Design review of the part shown in the three views and the two pictorial views. Dimensions are in mm from the part's minimum x, y and z. A direction names the side the tool comes from. Give positions to 0.01 mm unless a question says otherwise; leave off trailing zeros. Loops run counter-clockwise (first coordinate to the right, second up) from the corner with the lowest first, then second, coordinate; pieces in that order, holes last.
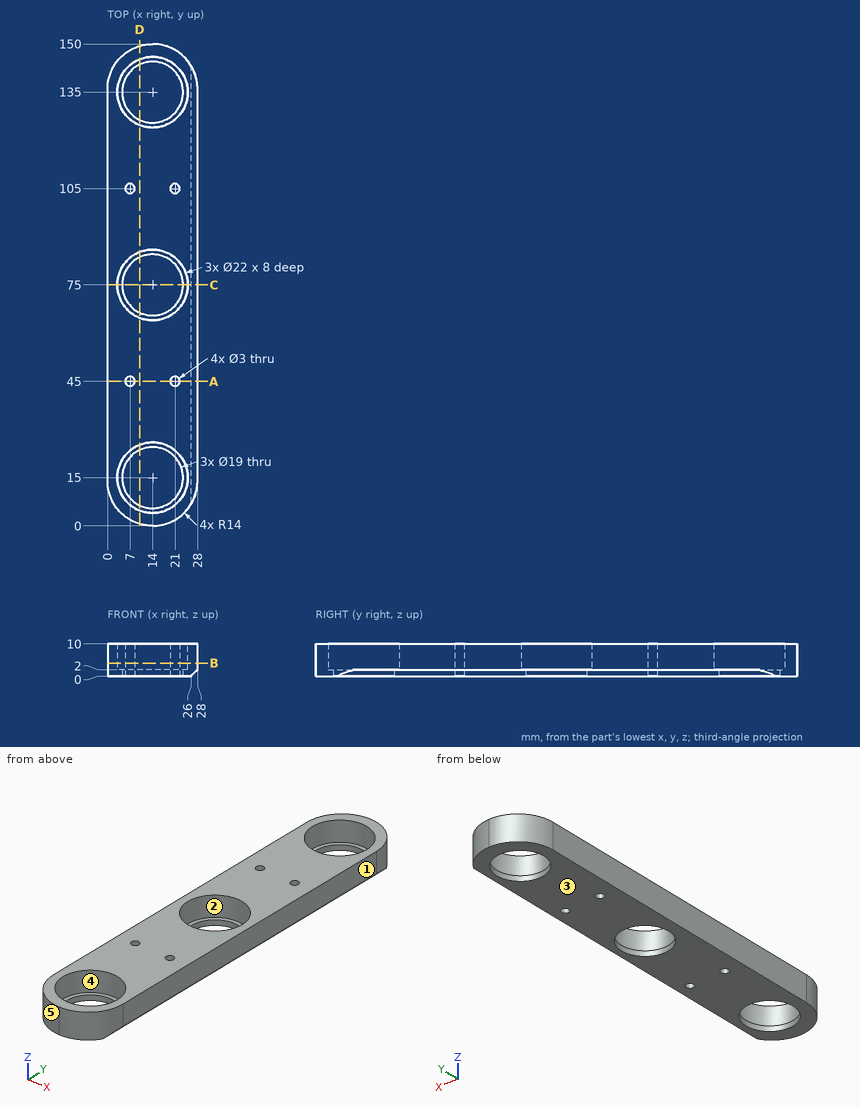
Q1. For probe 1 along X at (y, z) = (45, 6.25); probe 2 along Y at (x, z) = (14, 0.6); probe 3 along Y at (x, z) = (7, 4) (1 decimal), list the stretches that pass through material, from the lowest coordinate up.
Answers:
probe 1: x = 0 to 5.5, 8.5 to 19.5, 22.5 to 28
probe 2: y = 0 to 5.5, 24.5 to 65.5, 84.5 to 125.5, 144.5 to 150
probe 3: y = 1.9 to 6.5, 23.5 to 43.5, 46.5 to 66.5, 83.5 to 103.5, 106.5 to 126.5, 143.5 to 148.1
Q2. Consider section C-C on y = 75. Give the boundary of the cut face in (x, z).
Answers:
outline: (0, 0) - (4.5, 0) - (4.5, 2) - (3, 2) - (3, 10) - (0, 10) - close; (23.5, 0) - (26, 0) - (28, 2) - (28, 10) - (25, 10) - (25, 2) - (23.5, 2) - close
Q3. Consider section B-B on z = 4. Count the separate pieces of the cut face and the enclosed holes in it, plus the area to 3 significant figures.
Answers:
separate pieces: 1
enclosed holes: 7
area: 2,860 mm2
Q4. Consider section A-A on y = 45. Give the boundary of the cut face in (x, z).
Answers:
outline: (0, 0) - (5.5, 0) - (5.5, 10) - (0, 10) - close; (8.5, 0) - (19.5, 0) - (19.5, 10) - (8.5, 10) - close; (22.5, 0) - (26, 0) - (28, 2) - (28, 10) - (22.5, 10) - close
Q5. Mouldability with a two-part tool opening along X and no side actions: class the marked faces 3, 4 and 5 as +X half, -X half, draft (parallel to the pull), parting line (faces both ways), or undercut.
Answers:
face 3: draft
face 4: undercut
face 5: -X half
Q6. Machinability: for the marked faces 1 and 2, which of the approach directions +Z, -Z, +X, -X, +Y, -Y give a long, thin tool a straight path to every point of the face, cutting with its end or side? Answer none if there is none.
Answers:
face 1: +Z, -Z, +X, +Y, -Y
face 2: +Z
Q7. For pin 1 Ø1.5 at (x, z) = (24.5, 5.5) entering from +Y; pin 2 Ø1 at (x, z) = (24, 5) entering from -Y, all flat-tipped, find the tip position at first contact; note any pin that passes through.
Answers:
pin 1: stops at y = 146.05
pin 2: stops at y = 3.72
Q8. Consider section D-D on x = 10. Give the boundary of the cut face in (y, z).
Answers:
outline: (0.58, 0) - (6.38, 0) - (6.38, 2) - (4.75, 2) - (4.75, 10) - (0.58, 10) - close; (23.62, 0) - (66.38, 0) - (66.38, 2) - (64.75, 2) - (64.75, 10) - (25.25, 10) - (25.25, 2) - (23.62, 2) - close; (83.62, 0) - (126.38, 0) - (126.38, 2) - (124.75, 2) - (124.75, 10) - (85.25, 10) - (85.25, 2) - (83.62, 2) - close; (143.62, 0) - (149.42, 0) - (149.42, 10) - (145.25, 10) - (145.25, 2) - (143.62, 2) - close
